from build123d import *

# Parameters (mm, degrees)
CROQUIS1_W              = 25
CROQUIS1_H              = 50
SALIENTE_EXTRUIR1_DEPTH = 10
CROQUIS2_W              = 10
CROQUIS2_H              = 50
SALIENTE_EXTRUIR2_DEPTH = 40
CROQUIS3_W              = 8
CROQUIS3_H              = 42
CORTAR_EXTRUIR1_DEPTH   = 4
REDONDEO1_R             = 3
CROQUIS4_W              = 4.1
CROQUIS4_H              = 50
CORTAR_EXTRUIR2_DEPTH   = 4
CROQUIS5_R              = 3
CORTAR_EXTRUIR3_DEPTH   = 3.5
CORTAR_EXTRUIR4_START   = -4
CORTAR_EXTRUIR4_DEPTH   = 4
REDONDEO2_R             = 3
CROQUIS7_R              = 11.5
CORTAR_EXTRUIR5_DEPTH   = 15


with BuildPart() as part:
    # Croquis1 → Saliente-Extruir1 (new body)
    with BuildSketch(Plane(origin=(0, 0, 0), x_dir=(1, 0, 0), z_dir=(0, 1, 0))):
        with Locations((12.5, 25)):
            Rectangle(CROQUIS1_W, CROQUIS1_H)
    extrude(amount=SALIENTE_EXTRUIR1_DEPTH)

    # Croquis2 → Saliente-Extruir2 (add)
    with BuildSketch(Plane(origin=(0, 10, 0), x_dir=(1, 0, 0), z_dir=(0, 1, 0))):
        with Locations((12.5, 25)):
            Rectangle(CROQUIS2_W, CROQUIS2_H)
    extrude(amount=SALIENTE_EXTRUIR2_DEPTH)

    # Croquis3 → Cortar-Extruir1 (cut)
    with BuildSketch(Plane(origin=(0, 50, 0), x_dir=(1, 0, 0), z_dir=(0, 1, 0))):
        with Locations((11.5, 25)):
            Rectangle(CROQUIS3_W, CROQUIS3_H)
    extrude(amount=-CORTAR_EXTRUIR1_DEPTH, mode=Mode.SUBTRACT)

    # Redondeo1
    redondeo1_edges = [part.edges().sort_by_distance(p)[0] for p in [
        (15.5, 48, -46),
        (15.5, 48, -4),
    ]]
    fillet(redondeo1_edges, radius=REDONDEO1_R)

    # Croquis4 → Cortar-Extruir2 (cut)
    with BuildSketch(Plane(origin=(0, 50, 0), x_dir=(1, 0, 0), z_dir=(0, 1, 0))):
        with Locations((9.55, 25)):
            Rectangle(CROQUIS4_W, CROQUIS4_H)
    extrude(amount=-CORTAR_EXTRUIR2_DEPTH, mode=Mode.SUBTRACT)

    # Croquis5 → Cortar-Extruir3 (cut)
    with BuildSketch(Plane(origin=(0, 46, 0), x_dir=(1, 0, 0), z_dir=(0, 1, 0))):
        with Locations((9.5, 9.5)):
            Circle(CROQUIS5_R)
        with Locations((9.5, 40.5)):
            Circle(CROQUIS5_R)
    extrude(amount=-CORTAR_EXTRUIR3_DEPTH, mode=Mode.SUBTRACT)

    # Croquis6 → Cortar-Extruir4 (cut)
    with BuildSketch(Plane(origin=(0, 50, 0), x_dir=(1, 0, 0), z_dir=(0, 1, 0)).offset(CORTAR_EXTRUIR4_START)):
        with BuildLine():
            Line((11.6, 4), (12.5, 4))
            ThreePointArc((12.5, 4), (14.621320344, 4.878679656), (15.5, 7))
            Line((15.5, 7), (15.5, 43))
            ThreePointArc((15.5, 43), (14.621320344, 45.121320344), (12.5, 46))
            Line((12.5, 46), (11.6, 46))
            Line((11.6, 46), (11.6, 50))
            Line((11.6, 50), (11.75, 50))
            Line((11.75, 50), (11.75, 46.15))
            Line((11.75, 46.15), (12.5, 46.15))
            ThreePointArc((12.5, 46.15), (14.727386361, 45.227386361), (15.65, 43))
            Line((15.65, 43), (15.65, 7))
            ThreePointArc((15.65, 7), (14.727386361, 4.772613639), (12.5, 3.85))
            Line((12.5, 3.85), (11.75, 3.85))
            Line((11.75, 3.85), (11.75, 0))
            Line((11.75, 0), (11.6, 0))
            Line((11.6, 0), (11.6, 4))
        make_face()
    extrude(amount=CORTAR_EXTRUIR4_DEPTH, mode=Mode.SUBTRACT)

    # Redondeo2
    redondeo2_edges = [part.edges().sort_by_distance(p)[0] for p in [
        (7.5, 10, -25),
        (17.5, 10, -25),
        (0, 5, -50),
        (25, 5, -50),
        (25, 5, 0),
        (0, 5, 0),
    ]]
    fillet(redondeo2_edges, radius=REDONDEO2_R)

    # Croquis7 → Cortar-Extruir5 (cut)
    with BuildSketch(Plane.XZ):
        with Locations((-6, -25)):
            Circle(CROQUIS7_R)
    extrude(amount=-CORTAR_EXTRUIR5_DEPTH, mode=Mode.SUBTRACT)


solid = part.part
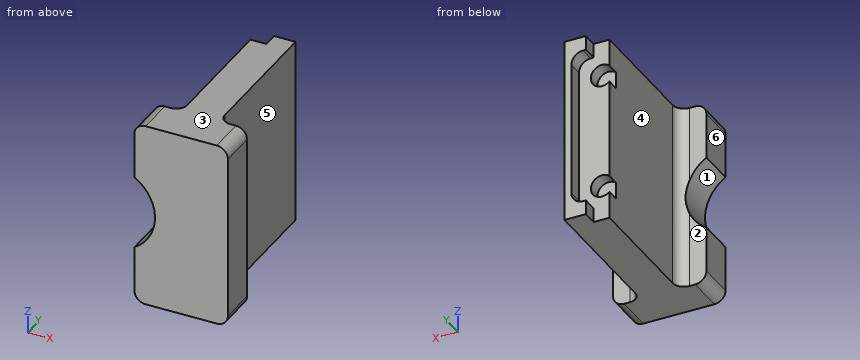
Can you work these out from the model? Positions are in its coordinate system, mm. Face numbers are marked on the shaded views. A direction names the side the tool comes from. Round coordinates to 2 decimals unless told otherwise and drop trailing zeros. Loops run counter-clockwise (first coordinate to the right, second up) from the corner with the lowest first, then second, coordinate; pieces in that order, holes last. Notation, with made-up numbers: (66.25, 83) - (94.25, 83) arc R17 ccw to (94.25, 100) - close; hole circle Ø1 at (13.5, 67.5). An arc over 180 degrees is marked (long way). Answer in a Markdown table with one row per item. Add a question column.
Q1. I want a section at B-B on z = -9.5. List the corners of the cut face in (x, y) for me.
Q2. I want a section at C-C on x = 1.75. List the corners of the cut face in (y, z) for me, and give its area (3 significant figures).
Q3. We'd pull the mould along Z, two halves only. Please class the marked faces 1, 2 and 3: pulls with the +Z half, pulls with the -Z half, needs draft (parallel to the pull), parting line crosses it, or undercut.
Q4. I want a section at D-D on y = 30.5. List the corners of the cut face in (x, z) for me.
Q5. I want a section at A-A on x = 9.5. List the corners of the cut face in (y, z) for me, and give its area (3 significant figures).
Q6. For pin 1 Ø0.8 at (x, y) = (12, 47.5) entering from +Z; pin 2 Ø6.5 at (x, z) = (11, -20) entering from +Y; pin 3 Ø5 at (y, z) = (26.5, -23) entering from -X; pin 4 Ø2.5 at (x, z) = (3.5, -7) entering from +Y, each with a flat end and sliding along its axis, tell me the tip position at first contact or that it passes through.
Q7. I need wall thicknesses on L1, parallel to Z at x = 9.5, y = 44; L2, parallel to X at y = 36.5, z = -45; L3, parallel to Y at x = 10, z = -4. Which ranges of each line are inside material? Lowest first, please.
Q8. Which directions (+Z, -Z, +X, -X, +Y, -Y) give clear straight access to the entire face, cutting with the end or side of a thin tool? Please do the marked faces 4, 5 and 6.
A:
| question | item | result |
|---|---|---|
| 1 | outline | (0, 0) - (25, 0) - (25, 10) - (20.5, 10) arc R3 cw to (17.5, 13) - (17.5, 50) - (15.65, 50) - (15.65, 46) - (12.5, 46) - (12.5, 42.5) - (7.5, 42.5) - (7.5, 13) arc R3 cw to (4.5, 10) - (0, 10) - close |
| 2 | outline | (0, -49.73) - (10, -49.73) - (10, -33.5) - (0, -33.5) - close; (0, -16.5) - (10, -16.5) - (10, -0.27) - (0, -0.27) - close |
| 2 | area | 325 mm^2 |
| 3 | face 1 | undercut |
| 3 | face 2 | needs draft |
| 3 | face 3 | pulls with the +Z half |
| 4 | outline | (7.5, -50) - (17.5, -50) - (17.5, 0) - (7.5, 0) - close |
| 5 | outline | (0, -50) - (46, -50) - (46, -43.5) - (42.5, -43.5) - (42.5, -37.5) - (46, -37.5) - (46, -12.5) - (42.5, -12.5) - (42.5, -6.5) - (46, -6.5) - (46, 0) - (0, 0) - close |
| 5 | area | 2,260 mm^2 |
| 6 | pin 1 | z = 0 |
| 6 | pin 2 | y = 46 |
| 6 | pin 3 | x = 7.5 |
| 6 | pin 4 | y = 10.01 |
| 7 | L1 | -50 to -43.5, -37.5 to -12.5, -6.5 to 0 |
| 7 | L2 | 7.5 to 17.5 |
| 7 | L3 | 0 to 46 |
| 8 | face 4 | +Z, -Z, -X, +Y |
| 8 | face 5 | +Z, -Z, +X, +Y |
| 8 | face 6 | +Z, -Z, -X, +Y, -Y |
